Source: CAD feature listing. Evaluate the final solid. Frame: model axes, mm. A direction names the side the tool comes from. Give positions to 0.01 mm unless a question says otherwise; leave off trailing zeros. Order: outer loops, then holes, each group sorted by start corner. A loop starts at its lowest first (then second) coordinate and runs counter-clockwise, first axis right, second up. Notation, with made-up numbers: (59.5, 7.5) -> (79.5, 7.5) arc R36 ccw to (79.5, 44.5) -> close; hole circle Ø4 at (-13, 9). An arc over 180 degrees is marked (long way). Answer in a Markdown table with one row per item.
```python
from build123d import *

# Parameters (mm, degrees)
BOSS_EXTRUDE1_DEPTH = 10.16
FILLET1_R           = 2.54
SKETCH2_R           = 3.302
CUT_EXTRUDE1_DEPTH  = 10.16
FILLET3_R           = 2.54
BOSS_EXTRUDE2_START = -0.524037
SKETCH4_W           = 12.7
SKETCH4_H           = 10.16
BOSS_EXTRUDE2_DEPTH = 0.524037
SKETCH4_2_W         = 12.7
SKETCH4_2_H         = 10.16
BOSS_EXTRUDE3_DEPTH = 6.477
FILLET4_R           = 3.175
SKETCH5_R           = 3.175
CUT_EXTRUDE2_DEPTH  = 3.81
SKETCH7_R           = 1.905
CUT_EXTRUDE3_DEPTH  = 42.402


with BuildPart() as part:
    # Sketch1 → Boss-Extrude1 (new body)
    with BuildSketch(Plane(origin=(0, 0, 0), x_dir=(1, 0, 0), z_dir=(0, 1, 0))):
        with BuildLine():
            Line((-54.61, 0), (-54.61, -3.175))
            Line((-54.61, -3.175), (-38.60465775, -3.175))
            ThreePointArc((-38.60465775, -3.175), (0, -38.735), (38.60465775, -3.175))
            Line((38.60465775, -3.175), (54.61, -3.175))
            Line((54.61, -3.175), (54.61, 0))
            Line((54.61, 0), (35.56, 0))
            ThreePointArc((35.56, 0), (0, -35.56), (-35.56, 0))
            Line((-35.56, 0), (-54.61, 0))
        make_face()
    extrude(amount=BOSS_EXTRUDE1_DEPTH)

    # Fillet1
    fillet1_edges = [part.edges().sort_by_distance(p)[0] for p in [
        (38.60465775, 5.08, 3.175),
        (-38.60465775, 5.08, 3.175),
    ]]
    fillet(fillet1_edges, radius=FILLET1_R)

    # Sketch2 → Cut-Extrude1 (cut)
    with BuildSketch(Plane.XY.offset(3.175)):
        with Locations((-47.743715713, 5.08)):
            Circle(SKETCH2_R)
        with Locations((47.743715713, 5.08)):
            Circle(SKETCH2_R)
    extrude(amount=-CUT_EXTRUDE1_DEPTH, mode=Mode.SUBTRACT)

    # Fillet3
    fillet3_edges = [part.edges().sort_by_distance(p)[0] for p in [
        (54.61, 5.08, 3.175),
        (-54.61, 5.08, 3.175),
    ]]
    fillet(fillet3_edges, radius=FILLET3_R)

    # Sketch4 → Boss-Extrude2 (add)
    with BuildSketch(Plane.XY.offset(38.735).offset(BOSS_EXTRUDE2_START)):
        with Locations((0, 5.08)):
            Rectangle(SKETCH4_W, SKETCH4_H)
    extrude(amount=BOSS_EXTRUDE2_DEPTH)

    # Sketch4_2 → Boss-Extrude3 (add)
    with BuildSketch(Plane.XY.offset(38.735)):
        with Locations((0, 5.08)):
            Rectangle(SKETCH4_2_W, SKETCH4_2_H)
    extrude(amount=BOSS_EXTRUDE3_DEPTH)

    # Fillet4
    fillet4_edges = [part.edges().sort_by_distance(p)[0] for p in [
        (6.35, 5.08, 38.210963),
        (-6.35, 5.08, 38.210963),
    ]]
    fillet(fillet4_edges, radius=FILLET4_R)

    # Sketch5 → Cut-Extrude2 (cut)
    with BuildSketch(Plane.XY.offset(45.212)):
        with Locations((0, 5.08)):
            Circle(SKETCH5_R)
    extrude(amount=-CUT_EXTRUDE2_DEPTH, mode=Mode.SUBTRACT)

    # Sketch7 → Cut-Extrude3 (cut, through all)
    with BuildSketch(Plane.XY.offset(41.402)):
        with Locations((0, 5.08)):
            Circle(SKETCH7_R)
    extrude(amount=-CUT_EXTRUDE3_DEPTH, mode=Mode.SUBTRACT)


solid = part.part
```
(1) Section query C-C (z = 32.5). Return the cut outline in (x, y), plus the area to 3 significant figures.
A:
| item | result |
|---|---|
| outline | (-21.07, 0) -> (-14.43, 0) -> (-14.43, 10.16) -> (-21.07, 10.16) -> close; (14.43, 0) -> (21.07, 0) -> (21.07, 10.16) -> (14.43, 10.16) -> close |
| area | 135 mm^2 |
(2) Access query for faces 5 (the cylindrical face through (0.78, 2.75, 35.55)), 6 (the cylindrical face through (-0.69, 1.98, 43.33)), 7 (the flat face through (6.35, 5, 43)). Directions: +Z, -Z, +X, -X, +Y, -Y. A direction counts if a zero-diameter tool reaches every point of the face in a straight line with its end or side. Return the directions, or none.
A:
| item | result |
|---|---|
| face 5 | -Z, +Y, -Y |
| face 6 | +Z |
| face 7 | +Z, +X, +Y, -Y |
(3) Section query D-D (z = 24). Return the cut outline in (x, y).
A:
| item | result |
|---|---|
| outline | (-30.4, 0) -> (-26.24, 0) -> (-26.24, 10.16) -> (-30.4, 10.16) -> close; (26.24, 0) -> (30.4, 0) -> (30.4, 10.16) -> (26.24, 10.16) -> close |
(4) Section query A-A (x = 0). Return the cut outline in (y, z) (3 decimals).
A:
| item | result |
|---|---|
| outline | (0, 35.56) -> (3.175, 35.56) -> (3.175, 41.402) -> (1.905, 41.402) -> (1.905, 45.212) -> (0, 45.212) -> close; (6.985, 35.56) -> (10.16, 35.56) -> (10.16, 45.212) -> (8.255, 45.212) -> (8.255, 41.402) -> (6.985, 41.402) -> close |
(5) Pull-direction query (Y, two-part tool) for faces 1 (the flat face through (-6.35, 5, 43)), 2 (the flat face through (0, 3, 41.402)), 3 (the flat face through (0, 10.16, 36)), 4 (the cylindrical face through (-51.043, 5.225, 1.61)); classes: +Y half, -Y half, draft (parallel to the pull), parting line (faces both ways), or undercut.
A:
| item | result |
|---|---|
| face 1 | draft |
| face 2 | undercut |
| face 3 | +Y half |
| face 4 | undercut |
(6) Section query B-B (y = 5.08). Give the number of separate pieces and of enclosed holes in the cut face, plus the area to 3 significant figures.
A:
| item | result |
|---|---|
| separate pieces | 4 |
| enclosed holes | 0 |
| area | 470 mm^2 |
(7) First-contact query: pin 1 Ø2 at (y, z) = (3.5, 43.5) entering from +X; pin 2 Ø4 at (x, y) = (47.74, 5.08) entering from -Z; pin 3 Ø3 at (x, y) = (-15.5, 9) entering from +Z; pin 4 Ø3 at (x, y) = (-44.5, 5.5) entering from +Z (3 decimals). Flat tips, straight axial feed; report the tip coordinate or a pass-through.
A:
| item | result |
|---|---|
| pin 1 | stops at x = 6.35 |
| pin 2 | passes through |
| pin 3 | stops at z = 36.12 |
| pin 4 | stops at z = 3.175 |
(8) Ray query, probe 1 along Y at (x, z) = (0, 38) (3 decimals); probe 2 along Z at (x, y) = (43, 1.5) (3 decimals); probe 3 along X at (y, z) = (6.75, 20.5). Return the intervals inside material, ascending.
A:
| item | result |
|---|---|
| probe 1 | y = 0 to 3.175, 6.985 to 10.16 |
| probe 2 | z = 0 to 3.175 |
| probe 3 | x = -32.87 to -29.06, 29.06 to 32.87 |
